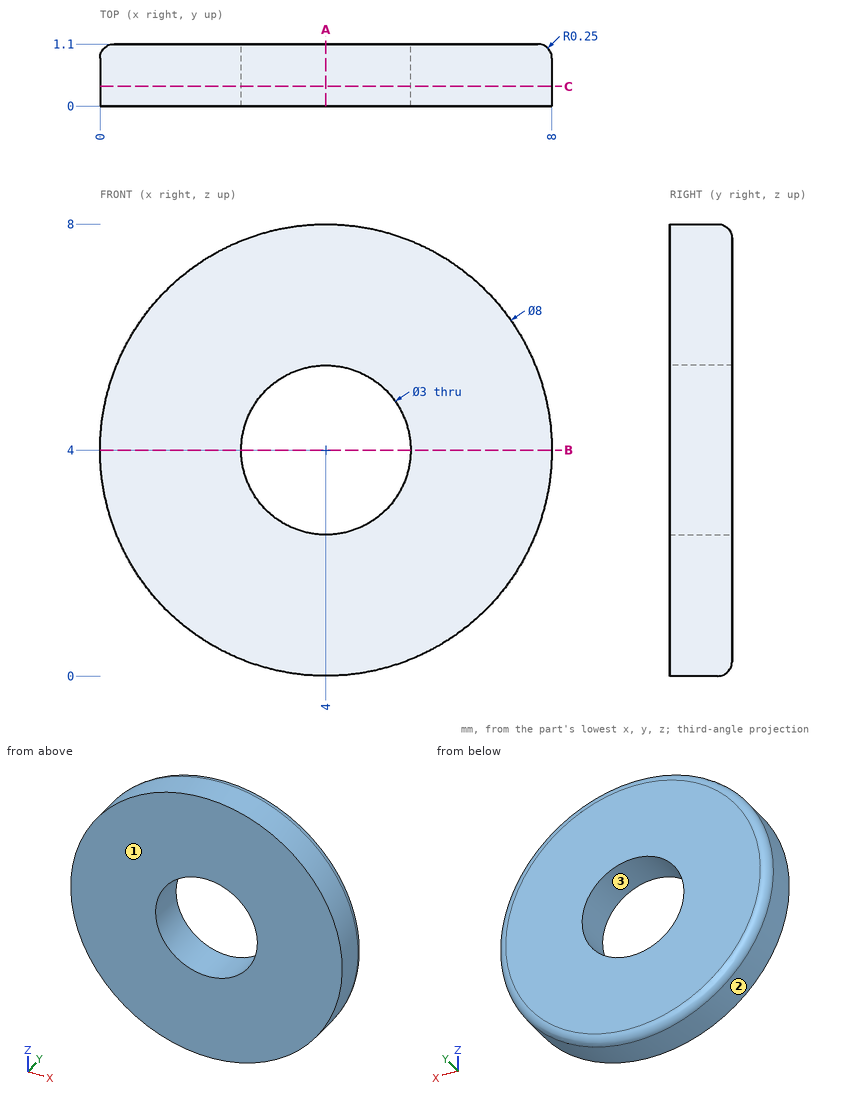
Study the drawing (mm; zero at the part's minimum x, y, z) and answer. Coordinates: 2 decimals unless noted, no trailing zeros. Write each loop counter-clockwise with the first axis right and the second up, starting at its lowest first coordinate (ties: lowest second). Pieces come first, ordered by that corner, then holes.
Q1. A cutting plane is placed at C-C, the plane y = 0.35. Give the vertices of the cut face in (x, z).
Q2. A cutting plane is placed at A-A, the plane x = 4. Give the vertices of the cut face in (y, z).
Q3. Determine the mould class of the marked faces 1, 2 and 3 for opening direction Z: released by +Z, released by -Z, zero draft, split by the parting line, or undercut.
Q4. A cutting plane is placed at B-B, the plane z = 4. Give the vertices of the cut face in (x, y).
Q5. Find the intervals of material crossed by line 1 (X direction, y = 0.65, z = 4); line 2 (Z direction, x = 4.5, y = 0.7); line 3 (Z direction, x = 4.75, y = 0.8), in increasing order.
Findings below:
1. outline: circle Ø8 at (4, 4); hole circle Ø3 at (4, 4)
2. outline: (0, 0) - (0.85, 0) arc R0.25 ccw to (1.1, 0.25) - (1.1, 2.5) - (0, 2.5) - close; (0, 5.5) - (1.1, 5.5) - (1.1, 7.75) arc R0.25 ccw to (0.85, 8) - (0, 8) - close
3. face 1: zero draft
3. face 2: split by the parting line
3. face 3: undercut
4. outline: (0, 0) - (2.5, 0) - (2.5, 1.1) - (0.25, 1.1) arc R0.25 ccw to (0, 0.85) - close; (5.5, 0) - (8, 0) - (8, 0.85) arc R0.25 ccw to (7.75, 1.1) - (5.5, 1.1) - close
5. line 1: x = 0 to 2.5, 5.5 to 8
5. line 2: z = 0.03 to 2.59, 5.41 to 7.97
5. line 3: z = 0.07 to 2.7, 5.3 to 7.93
